from build123d import *

# Parameters (mm, degrees)
F0_R      = 17
F1_DEPTH  = 5
F2_R      = 14
F3_DEPTH  = 15
F4_R      = 18.5
F5_DEPTH  = 10
F6_R      = 16.5
F7_DEPTH  = 35
F8_R      = 18.5
F9_DEPTH  = 10
F10_R     = 16.5
F11_DEPTH = 2
F12_R     = 18.5
F13_DEPTH = 3
F14_R     = 15
F15_DEPTH = 5
F16_R     = 11.5
F17_DEPTH = 136.4


with BuildPart() as f1:
    # F0 (on Front) → F1 (new body)
    with BuildSketch(Plane.XZ):
        Circle(F0_R)
    extrude(amount=F1_DEPTH)

    # F2 (on face) → F3 (join)
    with BuildSketch(Plane.XZ.offset(5)):
        Circle(F2_R)
    extrude(amount=F3_DEPTH)

    # F4 (on Front) → F5 (join)
    with BuildSketch(Plane.XZ):
        Circle(F4_R)
    extrude(amount=-F5_DEPTH)

    # F6 (on Front) → F7 (join)
    with BuildSketch(Plane.XZ):
        Circle(F6_R)
    extrude(amount=-F7_DEPTH)

    # F8 (on face) → F9 (join)
    with BuildSketch(Plane(origin=(0, 35, 0), x_dir=(-1, 0, 0), z_dir=(0, 1, 0))):
        Circle(F8_R)
    extrude(amount=F9_DEPTH)

    # F10 (on face) → F11 (join)
    with BuildSketch(Plane(origin=(0, 45, 0), x_dir=(-1, 0, 0), z_dir=(0, 1, 0))):
        Circle(F10_R)
    extrude(amount=F11_DEPTH)

    # F12 (on face) → F13 (join)
    with BuildSketch(Plane(origin=(0, 47, 0), x_dir=(-1, 0, 0), z_dir=(0, 1, 0))):
        Circle(F12_R)
    extrude(amount=F13_DEPTH)

    # F14 (on face) → F15 (join)
    with BuildSketch(Plane(origin=(0, 50, 0), x_dir=(-1, 0, 0), z_dir=(0, 1, 0))):
        Circle(F14_R)
    extrude(amount=F15_DEPTH)

    # F16 (on face) → F17 (cut)
    with BuildSketch(Plane(origin=(0, 55, 0), x_dir=(-1, 0, 0), z_dir=(0, 1, 0))):
        Circle(F16_R)
    extrude(amount=-F17_DEPTH, mode=Mode.SUBTRACT)


solid = f1.part
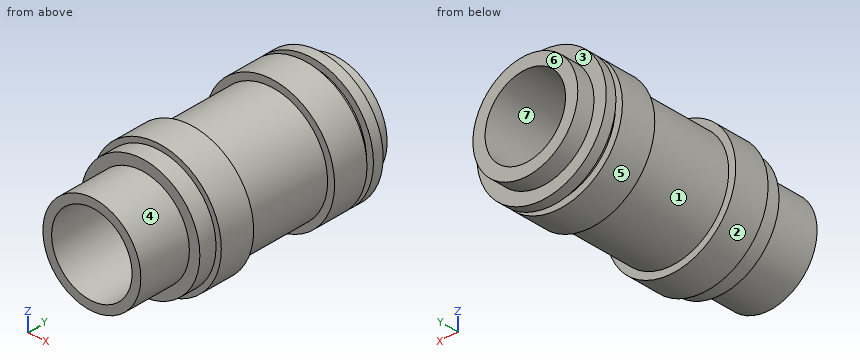
Source: CAD feature listing. Evaluate the final solid. Frame: model axes, mm. Face numbers are marked on the shaded views. A direction names the side the tool comes from. Round coordinates to 2 decimals unless told otherwise and drop trailing zeros. Loops run counter-clockwise (first coordinate to the right, second up) from the corner with the lowest first, then second, coordinate; pieces in that order, holes last. Notation, with made-up numbers: (45.5, 74) -> (92.5, 74) arc R7 ccw to (92.5, 86) -> close; hole circle Ø5 at (-31.5, 52). An arc over 180 degrees is marked (long way). Answer as a JSON object with one key per item and string values. Group by question number.
Q1. Contact query for flat-ended pins moving along their axis: P1, Ø4, axis at x = -1.5, y = -9.5, coming from the -Z side; P2, Ø5, axis at x = -8, y = 27, coming from the -Z side; P3, Ø10, axis at x = -9, y = 43, coming from the +Z side. Output: stop coordinate, or through.
Q2. Ray query, line 1 (Y direction, x = 6.5, z = 16); line 2 (Z direction, x = 0, y = 3); line 3 (Z direction, x = 0, y = 22). Return the intervals inside material, ascending. Write a range as from..to.
Q3. Access query for the marked faces 1, 2, 3 and 4. Directions: +Z, -Z, +X, -X, +Y, -Y. A direction counts if a zero-diameter tool reaches every point of the face in a straight line with its end or side. Return the directions, or none.
Q4. Section query B-B (y = -10). Output: boundary loops of the cut face in (x, z).
Q5. Section query A-A (y = 41). Output: boundary loops of the cut face in (x, z).
Q6. Mould query, pull axis X, two halves, no side actions, for the marked faces 5, 6 and 7. Classes: pulls with the +X half, pulls with the -X half, needs draft (parallel to the pull), parting line crosses it, or undercut.
Completed:
{
 "1": {"P1": "z = -14", "P2": "z = -15.56", "P3": "z = 18.06"},
 "2": {"line 1": "0..10, 35..45, 47..50", "line 2": "-18.5..-11.5, 11.5..18.5", "line 3": "-16.5..-11.5, 11.5..16.5"},
 "3": {"face 1": "none", "face 2": "+Y, -Y", "face 3": "+Y", "face 4": "-Y"},
 "4": {"outline": "circle Ø28 at (0, 0); hole circle Ø23 at (0, 0)"},
 "5": {"outline": "circle Ø37 at (0, 0); hole circle Ø23 at (0, 0)"},
 "6": {"face 5": "parting line crosses it", "face 6": "needs draft", "face 7": "undercut"}
}
